```python
from build123d import *

# Parameters (mm, degrees)
SKETCH1_R           = 41.91
BOSS_EXTRUDE1_DEPTH = 196.85
SKETCH6_R           = 19.05
BOSS_EXTRUDE4_DEPTH = 12.7
SHELL7_T            = -3.81
CUT_EXTRUDE2_REACH  = 225.888
SKETCH13_R          = 15.24
FILLET12_R          = 2.54


with BuildPart() as part:
    # Sketch1 → Boss-Extrude1 (new body)
    with BuildSketch(Plane(origin=(0, 0, 0), x_dir=(1, 0, 0), z_dir=(0, 1, 0))):
        with Locations(Location((0, 0, 0), (0, 0, 270))):
            Circle(SKETCH1_R)
    extrude(amount=BOSS_EXTRUDE1_DEPTH)

    # Shell7
    shell7_openings = [part.faces().sort_by_distance(p)[0] for p in [
        (0, 196.85, 0),
    ]]
    offset(amount=SHELL7_T, openings=shell7_openings, kind=Kind.INTERSECTION)



with BuildPart() as body_2:
    # Sketch6 → Boss-Extrude4 (new body)
    with BuildSketch(Plane(origin=(0, 203.2, 0), x_dir=(1, 0, 0), z_dir=(0, 1, 0))):
        with Locations(Location((0, 0, 0), (0, 0, 270))):
            Circle(SKETCH6_R)
    extrude(amount=BOSS_EXTRUDE4_DEPTH)


with BuildPart() as part_1:
    add(part.part)

    add(body_2.part)  # loft3 joins it to this body
    # loft up to a face of the part (loft3)
    loft([Face(Wire([part_1.edges().sort_by_distance((30.551075175, 196.85, -28.689369209))[0]])), Face(Wire([part_1.edges().sort_by_distance((-13.886852352, 203.2, -13.040622368))[0]]))])

    # Sketch13 → Cut-Extrude2 (cut, up to next)
    with BuildSketch(Plane(origin=(0, 215.9, 0), x_dir=(1, 0, 0), z_dir=(0, 1, 0)), mode=Mode.PRIVATE) as cut_extrude2_sk1:
        with Locations(Location((0, 0, 0), (0, 0, 270))):
            Circle(SKETCH13_R)
    cut_extrude2_tool1 = extrude(cut_extrude2_sk1.sketch, amount=-CUT_EXTRUDE2_REACH, mode=Mode.PRIVATE) & part_1.part
    add(cut_extrude2_tool1.solids().sort_by_distance((0, 215.9, 0))[0], mode=Mode.SUBTRACT)

    # Fillet12
    fillet12_edges = [part_1.edges().sort_by_distance(p)[0] for p in [
        (0, 215.9, -19.05),
        (0, 0, -41.91),
        (0, 196.85, -41.91),
        (0, 203.2, -19.05),
    ]]
    fillet(fillet12_edges, radius=FILLET12_R)


solid = part_1.part
```
Work out the finished part from the listing and answer in its coordinate system (mm). A direction names the side the tool comes from. Coordinates: 2 decimals unless noted, no trailing zeros. Order: outer loops, then holes, each group sorted by start corner. A loop starts at its lowest first (then second) coordinate and runs counter-clockwise, first axis right, second up. Notation, with made-up numbers: (-5.75, 19) - (51.25, 19) arc R29 cw to (51.25, 42) - close; hole circle Ø11 at (76, 59). An arc over 180 degrees is marked (long way). Answer as a JSON object with one key per item and string values.
1. Each of these flat-tipped pins is pushed along its axis until it touches: P1, Ø12, axis at x = -7.5, y = 161.5, coming from the +Z side; P2, Ø12, axis at y = 69, z = 15, coming from the -X side; P3, Ø4, axis at y = 102.5, z = 11, coming from the +X side. Where does it stop, or does it pass through?
Output values:
{"P1": "stops at z = 41.88", "P2": "stops at x = -40.93", "P3": "stops at x = 40.93"}
2. Find section A-A on y = 124. Determine the outline of the cut face in (x, z).
Output values:
{"outline": "circle Ø83.82 at (0, 0); hole circle Ø76.2 at (0, 0)"}
3. A tool of negligible diameter and unlimited length cuts with its end or side. For faces 5 (the face through (5.72, 209.19, 18.17)), 6 (the face through (-23.183, 98.979, -30.235)), 7 (the face through (-5, 215.9, 15)), from which of +Z, -Z, +X, -X, +Y, -Y can it reach the whole face along a straight path? Write none if from no direction.
Output values:
{"face 5": "+Y", "face 6": "none", "face 7": "+Z, -Z, +X, -X, +Y"}
4. The mould has two halves that part along Y. Classify faces 1 (the face through (1, 0, -1)), 2 (the face through (1, 3.81, -1)), 3 (the face through (1, 196.85, 16)), 4 (the face through (35.34, 97.38, 22.53)): +Y half, -Y half, draft (parallel to the pull), parting line (faces both ways), or undercut.
Output values:
{"face 1": "-Y half", "face 2": "undercut", "face 3": "undercut", "face 4": "draft"}
5. Consider line 1 (X direction, y = 207, z = 0); line 2 (Y direction, x = 33, z = -14). Determine where each line is inside the solid, lowest interval first.
Output values:
{"line 1": "x = -19.05 to -15.24, 15.24 to 19.05", "line 2": "y = 0 to 3.81, 196.85 to 198.53"}
